For this review, take the finished solid that the model builds, in its own axes (mm). A direction names the side the tool comes from. Give positions to 0.01 mm unless a question says otherwise; leave off trailing zeros. Use a Markdown table: item, result. Add a question column.
1) Machinability: for faces 4 (the face through (-7.245, -4.93, -4.183)), 5 (the face through (9.436, -4.93, -1.368)), 6 (the face through (6.422, -4.93, 5.389)), 7 (the face through (2.86, -4.93, 7.86)), which of the approach directions +Z, -Z, +X, -X, +Y, -Y give a long, thin tool a straight path to every point of the face, cutting with its end or side? Answer none if there is none.
2) Mouldability with a two-part tool opening along Z and no side actions: class faces 1 (the face through (0.68, -4.93, 7.72)), 2 (the face through (7.72, -4.93, 0.67)), 3 (the face through (-5, -4.9, -8.1)) as released by +Z, released by -Z, zero draft, split by the parting line, or undercut.
3) Wall thickness on L1, parallel to Z at x = 8, y = -3; L2, parallel to X at y = -0.5, z = 0.75; L3, parallel to Z at x = 5.25, y = -7: over which ranges is each line inside the solid? List them lowest first.
4) Clearance check with flat-ended pins moving along their axes: P1, Ø1.5, axis at x = 4, y = -5, coming from the +Z side; P2, Ø2, axis at x = -3, y = -5, coming from the -Z side; P3, Ø1.4, axis at x = -8, y = -6, coming from the -Z side. State where each tip first meets the part, or that it passes through.
```python
from build123d import *

# Parameters (mm, degrees)
F0_R     = 4
F1_DEPTH = 10


with BuildPart() as f1:
    # F0 (on Front) → F1 (new body)
    with BuildSketch(Plane.XZ):
        with BuildLine():
            Line((-1.562834, 8.86327), (-1.345773, 7.63226))
            ThreePointArc((-1.345773, 7.63226), (-2.005848, 7.485925), (-2.650656, 7.282618))
            Line((-2.650656, 7.282618), (-3.078181, 8.457234))
            ThreePointArc((-3.078181, 8.457234), (-3.540527, 8.860187), (-4.094507, 9.123322))
            Line((-4.094507, 9.123322), (-4.356972, 9.000933))
            ThreePointArc((-4.356972, 9.000933), (-4.51149, 8.407419), (-4.5, 7.794229))
            Line((-4.5, 7.794229), (-3.875, 6.711697))
            ThreePointArc((-3.875, 6.711697), (-4.445217, 6.348428), (-4.981604, 5.936844))
            Line((-4.981604, 5.936844), (-5.785088, 6.8944))
            ThreePointArc((-5.785088, 6.8944), (-6.357369, 7.114921), (-6.967938, 7.172715))
            Line((-6.967938, 7.172715), (-7.172715, 6.967938))
            ThreePointArc((-7.172715, 6.967938), (-7.114921, 6.357369), (-6.8944, 5.785088))
            Line((-6.8944, 5.785088), (-5.936844, 4.981604))
            ThreePointArc((-5.936844, 4.981604), (-6.348428, 4.445217), (-6.711697, 3.875))
            Line((-6.711697, 3.875), (-7.794229, 4.5))
            ThreePointArc((-7.794229, 4.5), (-8.407419, 4.51149), (-9.000933, 4.356972))
            Line((-9.000933, 4.356972), (-9.123322, 4.094507))
            ThreePointArc((-9.123322, 4.094507), (-8.860187, 3.540527), (-8.457234, 3.078181))
            Line((-8.457234, 3.078181), (-7.282618, 2.650656))
            ThreePointArc((-7.282618, 2.650656), (-7.485925, 2.005848), (-7.63226, 1.345773))
            Line((-7.63226, 1.345773), (-8.86327, 1.562834))
            ThreePointArc((-8.86327, 1.562834), (-9.44341, 1.363908), (-9.948283, 1.015714))
            Line((-9.948283, 1.015714), (-9.973523, 0.727218))
            ThreePointArc((-9.973523, 0.727218), (-9.536784, 0.296644), (-9, 0))
            Line((-9, 0), (-7.75, 0))
            ThreePointArc((-7.75, 0), (-7.720509, -0.675457), (-7.63226, -1.345773))
            Line((-7.63226, -1.345773), (-8.86327, -1.562834))
            ThreePointArc((-8.86327, -1.562834), (-9.340387, -1.948183), (-9.695722, -2.448054))
            Line((-9.695722, -2.448054), (-9.620769, -2.727784))
            ThreePointArc((-9.620769, -2.727784), (-9.063104, -2.983018), (-8.457234, -3.078181))
            Line((-8.457234, -3.078181), (-7.282618, -2.650656))
            ThreePointArc((-7.282618, -2.650656), (-7.023885, -3.275292), (-6.711697, -3.875))
            Line((-6.711697, -3.875), (-7.794229, -4.5))
            ThreePointArc((-7.794229, -4.5), (-8.110775, -5.025293), (-8.273715, -5.616551))
            Line((-8.273715, -5.616551), (-8.107608, -5.853776))
            ThreePointArc((-8.107608, -5.853776), (-7.496279, -5.902884), (-6.8944, -5.785088))
            Line((-6.8944, -5.785088), (-5.936844, -4.981604))
            ThreePointArc((-5.936844, -4.981604), (-5.480078, -5.480078), (-4.981604, -5.936844))
            Line((-4.981604, -5.936844), (-5.785088, -6.8944))
            ThreePointArc((-5.785088, -6.8944), (-5.902884, -7.496279), (-5.853776, -8.107608))
            Line((-5.853776, -8.107608), (-5.616551, -8.273715))
            ThreePointArc((-5.616551, -8.273715), (-5.025293, -8.110775), (-4.5, -7.794229))
            Line((-4.5, -7.794229), (-3.875, -6.711697))
            ThreePointArc((-3.875, -6.711697), (-3.275292, -7.023885), (-2.650656, -7.282618))
            Line((-2.650656, -7.282618), (-3.078181, -8.457234))
            ThreePointArc((-3.078181, -8.457234), (-2.983018, -9.063104), (-2.727784, -9.620769))
            Line((-2.727784, -9.620769), (-2.448054, -9.695722))
            ThreePointArc((-2.448054, -9.695722), (-1.948183, -9.340387), (-1.562834, -8.86327))
            Line((-1.562834, -8.86327), (-1.345773, -7.63226))
            ThreePointArc((-1.345773, -7.63226), (-0.675457, -7.720509), (0, -7.75))
            Line((0, -7.75), (0, -9))
            ThreePointArc((0, -9), (0.296644, -9.536784), (0.727218, -9.973523))
            Line((0.727218, -9.973523), (1.015714, -9.948283))
            ThreePointArc((1.015714, -9.948283), (1.363908, -9.44341), (1.562834, -8.86327))
            Line((1.562834, -8.86327), (1.345773, -7.63226))
            ThreePointArc((1.345773, -7.63226), (2.005848, -7.485925), (2.650656, -7.282618))
            Line((2.650656, -7.282618), (3.078181, -8.457234))
            ThreePointArc((3.078181, -8.457234), (3.540527, -8.860187), (4.094507, -9.123322))
            Line((4.094507, -9.123322), (4.356972, -9.000933))
            ThreePointArc((4.356972, -9.000933), (4.51149, -8.407419), (4.5, -7.794229))
            Line((4.5, -7.794229), (3.875, -6.711697))
            ThreePointArc((3.875, -6.711697), (4.445217, -6.348428), (4.981604, -5.936844))
            Line((4.981604, -5.936844), (5.785088, -6.8944))
            ThreePointArc((5.785088, -6.8944), (6.357369, -7.114921), (6.967938, -7.172715))
            Line((6.967938, -7.172715), (7.172715, -6.967938))
            ThreePointArc((7.172715, -6.967938), (7.114921, -6.357369), (6.8944, -5.785088))
            Line((6.8944, -5.785088), (5.936844, -4.981604))
            ThreePointArc((5.936844, -4.981604), (6.348428, -4.445217), (6.711697, -3.875))
            Line((6.711697, -3.875), (7.794229, -4.5))
            ThreePointArc((7.794229, -4.5), (8.407419, -4.51149), (9.000933, -4.356972))
            Line((9.000933, -4.356972), (9.123322, -4.094507))
            ThreePointArc((9.123322, -4.094507), (8.860187, -3.540527), (8.457234, -3.078181))
            Line((8.457234, -3.078181), (7.282618, -2.650656))
            ThreePointArc((7.282618, -2.650656), (7.485925, -2.005848), (7.63226, -1.345773))
            Line((7.63226, -1.345773), (8.86327, -1.562834))
            ThreePointArc((8.86327, -1.562834), (9.44341, -1.363908), (9.948283, -1.015714))
            Line((9.948283, -1.015714), (9.973523, -0.727218))
            ThreePointArc((9.973523, -0.727218), (9.536784, -0.296644), (9, 0))
            Line((9, 0), (7.75, 0))
            ThreePointArc((7.75, 0), (7.720509, 0.675457), (7.63226, 1.345773))
            Line((7.63226, 1.345773), (8.86327, 1.562834))
            ThreePointArc((8.86327, 1.562834), (9.340387, 1.948183), (9.695722, 2.448054))
            Line((9.695722, 2.448054), (9.620769, 2.727784))
            ThreePointArc((9.620769, 2.727784), (9.063104, 2.983018), (8.457234, 3.078181))
            Line((8.457234, 3.078181), (7.282618, 2.650656))
            ThreePointArc((7.282618, 2.650656), (7.023885, 3.275292), (6.711697, 3.875))
            Line((6.711697, 3.875), (7.794229, 4.5))
            ThreePointArc((7.794229, 4.5), (8.110775, 5.025293), (8.273715, 5.616551))
            Line((8.273715, 5.616551), (8.107608, 5.853776))
            ThreePointArc((8.107608, 5.853776), (7.496279, 5.902884), (6.8944, 5.785088))
            Line((6.8944, 5.785088), (5.936844, 4.981604))
            ThreePointArc((5.936844, 4.981604), (5.480078, 5.480078), (4.981604, 5.936844))
            Line((4.981604, 5.936844), (5.785088, 6.8944))
            ThreePointArc((5.785088, 6.8944), (5.902884, 7.496279), (5.853776, 8.107608))
            Line((5.853776, 8.107608), (5.616551, 8.273715))
            ThreePointArc((5.616551, 8.273715), (5.025293, 8.110775), (4.5, 7.794229))
            Line((4.5, 7.794229), (3.875, 6.711697))
            ThreePointArc((3.875, 6.711697), (3.275292, 7.023885), (2.650656, 7.282618))
            Line((2.650656, 7.282618), (3.078181, 8.457234))
            ThreePointArc((3.078181, 8.457234), (2.983018, 9.063104), (2.727784, 9.620769))
            Line((2.727784, 9.620769), (2.448054, 9.695722))
            ThreePointArc((2.448054, 9.695722), (1.948183, 9.340387), (1.562834, 8.86327))
            Line((1.562834, 8.86327), (1.345773, 7.63226))
            ThreePointArc((1.345773, 7.63226), (0.675457, 7.720509), (0, 7.75))
            Line((0, 7.75), (0, 9))
            ThreePointArc((0, 9), (-0.296644, 9.536784), (-0.727218, 9.973523))
            Line((-0.727218, 9.973523), (-1.015714, 9.948283))
            ThreePointArc((-1.015714, 9.948283), (-1.363908, 9.44341), (-1.562834, 8.86327))
        make_face()
        Circle(F0_R, mode=Mode.SUBTRACT)
    extrude(amount=F1_DEPTH)


solid = f1.part
```
Checked values:
| question | item | result |
|---|---|---|
| 1 | face 4 | -X, +Y, -Y |
| 1 | face 5 | +X, +Y, -Y |
| 1 | face 6 | +Z, +Y, -Y |
| 1 | face 7 | +Y, -Y |
| 2 | face 1 | released by +Z |
| 2 | face 2 | undercut |
| 2 | face 3 | released by -Z |
| 3 | L1 | -4.52 to -2.91, -1.41 to 0, 1.41 to 2.91, 4.8 to 5.87 |
| 3 | L2 | -9.97 to -3.93, 3.93 to 7.71 |
| 3 | L3 | -6.26 to 5.7, 6.26 to 8.19 |
| 4 | P1 | z = 7.97 |
| 4 | P2 | z = -9.7 |
| 4 | P3 | z = -5.91 |
